Answer from the drawing. Dimensions are ordinates in mm from the lowest x, y and z of the part. A direction names the side the tool comes from. Give positions to 0.01 mm unless a question says otherwise; leave off trailing zeros. Loops run counter-clockwise (first coordinate to the right, second up) from the corner with the lowest first, then second, coordinate; pieces in that order, holes last. Notation, with made-up numbers: (84.25, 17) - (134.25, 17) arc R5 ccw to (134.25, 25) - close; hole circle Ø10 at (-39, 63). An arc over 180 degrees is marked (long way). Answer as CSV lines item,"result". Start each with the question number.
1) Flat-ended cylindrical pins translate along their axes: pin 1 (4 mm diameter, centred on x = 5.5, z = 4, fed in from -Y); pin 2 (2.5 mm diameter, centred on x = 6.35, y = 3.175, fed in from -Z) (1 decimal); pin 3 (2 mm diameter, centred on y = 4, z = 2, fed in from +X). Find the tip coordinate at first contact, or state that the pin passes through.
2) For the marked faces 1 and 2, determine the directions among +Z, -Z, +X, -X, +Y, -Y from which every point of the face is accessible in a straight line to the end or side of a thin tool.
3) Find the intervals of material crossed by line 1 along X through (y, z) = (1.25, 4); line 2 along X through (y, z) = (2.25, 7.75) (1 decimal); line 3 along Z through (x, y) = (7.5, 5.5) (1 decimal), in increasing order.
4) A cutting plane is placed at D-D (y = 3.75). Determine the outline of the cut face in (x, z) (1 decimal).
5) For a pull along Z with two mould halves and no side action, classify the marked faces 3, 4, 5 and 6 as pulls with the +Z half, pulls with the -Z half, needs draft (parallel to the pull), parting line crosses it, or undercut.
6) A cutting plane is placed at B-B (z = 2.5). Determine the outline of the cut face in (x, y).
7) A cutting plane is placed at C-C (y = 5.5). Determine the outline of the cut face in (x, z) (1 decimal).
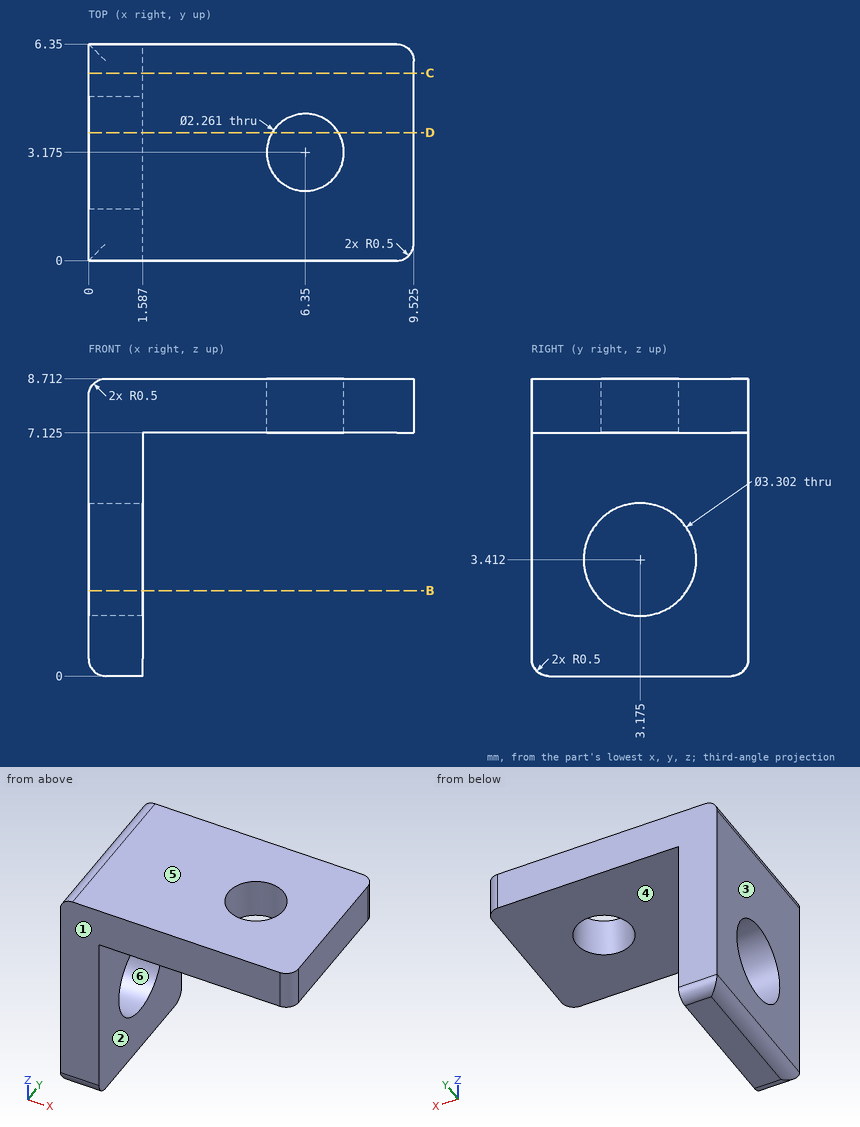
Ans:
1,pin 1,"through"
1,pin 2,"z = 7.1"
1,pin 3,"x = 1.59"
2,face 1,"+Z, -Z, +X, -X, -Y"
2,face 2,"-Z, +X, +Y, -Y"
3,line 1,"0 to 1.59"
3,line 2,"0 to 5.7, 7 to 9.5"
3,line 3,"7.1 to 8.7"
4,outline,"(0, 0.5) arc R0.5 ccw to (0.5, 0) - (1.6, 0) - (1.6, 1.9) - (0, 1.9) - close; (0, 5) - (1.6, 5) - (1.6, 7.1) - (5.4, 7.1) - (5.4, 8.7) - (0.5, 8.7) arc R0.5 ccw to (0, 8.2) - close; (7.3, 7.1) - (9.5, 7.1) - (9.5, 8.7) - (7.3, 8.7) - close"
5,face 3,"needs draft"
5,face 4,"pulls with the -Z half"
5,face 5,"pulls with the +Z half"
5,face 6,"undercut"
6,outline,"(0, 0) - (1.59, 0) - (1.59, 1.8) - (0, 1.8) - close; (0, 4.55) - (1.59, 4.55) - (1.59, 6.35) - (0, 6.35) - close"
7,outline,"(0, 0.5) arc R0.5 ccw to (0.5, 0) - (1.6, 0) - (1.6, 7.1) - (9.5, 7.1) - (9.5, 8.7) - (0.5, 8.7) arc R0.5 ccw to (0, 8.2) - close"
